```python
from build123d import *

# Parameters (mm, degrees)
BOSS_EXTRUDE1_DEPTH = 4
CIRPATTERN2_COUNT   = 5
CIRPATTERN2_ANGLE   = 180
BOSS_EXTRUDE3_DEPTH = 4


with BuildPart() as part:
    # Sketch1 → Boss-Extrude1 (new body)
    with BuildSketch(Plane(origin=(0, 0, 0), x_dir=(1, 0, 0), z_dir=(0, 1, 0))):
        with BuildLine():
            Line((0.25, 7.99381848), (-0.25, 7.99381848))
            ThreePointArc((-0.25, 7.99381848), (-0.831305349, 6.545394817), (-1, 4.99381848))
            Line((-1, 4.99381848), (1, 4.99381848))
            ThreePointArc((1, 4.99381848), (0.831305349, 6.545394817), (0.25, 7.99381848))
        make_face()
        with BuildLine():
            Line((0, 6.49381848), (0.843945674, 6.49381848))
            ThreePointArc((0.843945674, 6.49381848), (1.27002788, 5.491773836), (2, 4.683825681))
            Line((2, 4.683825681), (-2, 4.683825681))
            ThreePointArc((-2, 4.683825681), (-1.27002788, 5.491773836), (-0.843945674, 6.49381848))
            Line((-0.843945674, 6.49381848), (0, 6.49381848))
        make_face()
    boss_extrude1 = extrude(amount=BOSS_EXTRUDE1_DEPTH)

    # CirPattern2: Boss-Extrude1 ×5 about axis
    cirpattern2_axis = Axis((0, 0, 0), (0, -1, 0))
    for i in range(1, CIRPATTERN2_COUNT):
        add(boss_extrude1.rotate(cirpattern2_axis, i * CIRPATTERN2_ANGLE / (CIRPATTERN2_COUNT - 1)))

    # Sketch1<5> → Boss-Extrude3 (add)
    with BuildSketch(Plane(origin=(0, 0, 0), x_dir=(1, 0, 0), z_dir=(0, 1, 0))):
        with BuildLine():
            ThreePointArc((5.092958179, 0), (4.249949374, 2.806448526), (2, 4.683825681))
            Line((2, 4.683825681), (-2, 4.683825681))
            ThreePointArc((-2, 4.683825681), (-2.806448526, -4.249949374), (5.092958179, 0))
        make_face()
        with BuildLine():
            ThreePointArc((0.884943501, -2.15), (0.451040464, -2.280830441), (0, -2.325))
            ThreePointArc((0, -2.325), (-0.451040464, -2.280830441), (-0.884943501, -2.15))
            ThreePointArc((-0.884943501, -2.15), (-2.280830441, 0.451040464), (0, 2.325))
            ThreePointArc((0, 2.325), (1.644023266, 1.644023266), (2.325, 0))
            ThreePointArc((2.325, 0), (1.931724442, -1.293856901), (0.884943501, -2.15))
        make_face(mode=Mode.SUBTRACT)
    extrude(amount=BOSS_EXTRUDE3_DEPTH)


solid = part.part
```
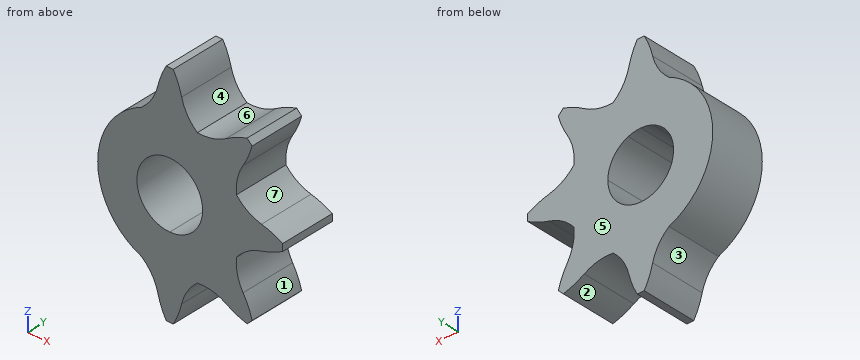
Can you work these out from the model? Positions are in its coordinate system, mm. Face numbers are marked on the shaded views. A direction names the side the tool comes from. Coordinates: 2 decimals unless noted, no trailing zeros. Loops run counter-clockwise (first coordinate to the right, second up) from the corner with the lowest first, then second, coordinate; pieces in that order, holes last. Notation, with made-up numbers: (79.25, 21) -> (111.25, 21) arc R20 ccw to (111.25, 49) -> close; hole circle Ø5 at (46.25, 77). An arc over 180 degrees is marked (long way). Put each result on its own line as item: value. Start each with the question number.
Q1. For the marked faces 1, 2, 3 and 4, which set-ups out of +Z, -Z, +X, -X, +Y, -Y let a thin tool reach every point of the face, with its end or its side?
Q2. Thinking about a two-plate mould opening in X: for the marked faces 5, 6 and 7, which applies, pulls with the +X half, pulls with the -X half, needs draft (parallel to the pull), parting line crosses it, or undercut?
Q3. I want a section at B-B (x = 1.75). Write out the boundary of the cut face in (y, z).
Q4. I want a section at D-D (x = -3.75). Write out the boundary of the cut face in (y, z), plus the area to 3 significant figures.
Q5. I'm going to push flat-ended pins straight in: P1, Ø1, axis at x = 0.5, y = 1, coming from the +Z side; P2, Ø1.5, axis at x = 6, y = 0.5, coming from the +Z side. Where does each tip first touch, or does it pass through?
Q6. I want a section at A-A (y = 1.55). Write out the boundary of the cut face in (x, z) (3 decimals), plus the area to 3 significant figures.
Q7. If I drill on line 1 (Z direction, x = 1.75, y = 2.6); line 2 (X direction, y = 2.65, z = -6.5); line 3 (X direction, y = 0.5, z = 2), over which ranges is the centre line in solid material (lowest first)? Write a range as [from, to].
Q8. I want a section at C-C (z = 5). Write out the boundary of the cut face in (x, y), plus the area to 3 significant figures.
Taken from the geometry:
1. face 1: +X, +Y, -Y
1. face 2: -Z, +Y, -Y
1. face 3: -Z, -X, +Y, -Y
1. face 4: +Z, +Y, -Y
2. face 5: needs draft
2. face 6: undercut
2. face 7: pulls with the +X half
3. outline: (0, -4.9) -> (4, -4.9) -> (4, -1.53) -> (0, -1.53) -> close; (0, 1.53) -> (4, 1.53) -> (4, 4.9) -> (0, 4.9) -> close
4. outline: (0, -3.45) -> (4, -3.45) -> (4, 3.45) -> (0, 3.45) -> close
4. area: 27.6 mm2
5. P1: stops at z = 7.99
5. P2: stops at z = 5.83
6. outline: (-2, -4.684) arc R3.288 cw to (-0.844, -6.494) arc R5.727 ccw to (-0.25, -7.994) -> (0.25, -7.994) arc R5.727 ccw to (0.844, -6.494) arc R3.288 cw to (1.955, -4.72) arc R3.288 cw to (3.995, -5.189) arc R5.727 ccw to (5.476, -5.829) -> (5.829, -5.476) arc R5.727 ccw to (5.189, -3.995) arc R3.288 cw to (4.72, -1.955) arc R3.288 cw to (6.494, -0.844) arc R5.727 ccw to (7.994, -0.25) -> (7.994, 0.25) arc R5.727 ccw to (6.494, 0.844) arc R3.288 cw to (4.72, 1.955) arc R3.288 cw to (5.189, 3.995) arc R5.727 ccw to (5.829, 5.476) -> (5.476, 5.829) arc R5.727 ccw to (3.995, 5.189) arc R3.288 cw to (1.955, 4.72) arc R3.288 cw to (0.844, 6.494) arc R5.727 ccw to (0.25, 7.994) -> (-0.25, 7.994) arc R5.727 ccw to (-0.844, 6.494) arc R3.288 cw to (-2, 4.684) arc R5.093 ccw to start; hole circle Ø4.65 at (0, 0)
6. area: 91.0 mm2
7. line 1: z = [-4.9, -1.53], [1.53, 4.9]
7. line 2: x = [-0.84, 0.84]
7. line 3: x = [-4.68, -1.19], [1.19, 4.72]
8. outline: (-1.65, 0) -> (1.65, 0) -> (1.65, 4) -> (-1.65, 4) -> close; (3.64, 0) -> (5.68, 0) -> (5.68, 4) -> (3.64, 4) -> close
8. area: 21.4 mm2
